```python
from build123d import *

# Parameters (mm, degrees)
SKETCH_1_W          = 120
SKETCH_1_H          = 65
EXTRUDE_1_DEPTH     = 2
EXTRUDE_2_DEPTH     = 2
SKETCH_3_R          = 2.1
CUT_EXTRUDE_1_DEPTH = 2
SKETCH_4_R          = 4
CUT_EXTRUDE_2_DEPTH = 70


with BuildPart() as part:
    # 草图1 → 凸台-拉伸1 (new body)
    with BuildSketch(Plane.XY):
        with Locations((24.994747839, 60.778264202)):
            Rectangle(SKETCH_1_W, SKETCH_1_H)
    extrude(amount=EXTRUDE_1_DEPTH)

    # 草图2 → 凸台-拉伸2 (add)
    with BuildSketch(Plane.XZ.offset(-28.278264202)):
        Polygon((-35.005252161, 2), (-35.005252161, 0), (-35.005252161, -5), (84.994747839, -28), (84.994747839, 2), align=None)
    extrude_2 = extrude(amount=EXTRUDE_2_DEPTH)

    # 镜向1: 凸台-拉伸2 across plane
    add(extrude_2.mirror(Plane.ZX.offset(60.778264202)))

    # 草图3 → 切除-拉伸1 (cut)
    with BuildSketch(Plane.XY.offset(2)):
        with Locations((-15.005252161, 80.778264202)):
            Circle(SKETCH_3_R)
        with Locations((4.994747839, 80.778264202)):
            Circle(SKETCH_3_R)
        with Locations((-15.005252161, 40.778264202)):
            Circle(SKETCH_3_R)
        with Locations((4.994747839, 40.778264202)):
            Circle(SKETCH_3_R)
    extrude(amount=-CUT_EXTRUDE_1_DEPTH, mode=Mode.SUBTRACT)

    # 草图4 → 切除-拉伸2 (cut)
    with BuildSketch(Plane(origin=(0, 26.278264202, 0), x_dir=(-1, 0, 0), z_dir=(0, -1, 0))):
        with Locations((-74.994747839, 8)):
            Circle(SKETCH_4_R)
    extrude(amount=-CUT_EXTRUDE_2_DEPTH, mode=Mode.SUBTRACT)


solid = part.part
```
Check sheet for the modelled part. Datum: model origin and axes. Units: mm. A direction names the side the tool comes from. Round coordinates to 2 decimals unless told otherwise and drop trailing zeros. Order: outer loops, then holes, each group sorted by start corner. A loop starts at its lowest first (then second) coordinate and runs counter-clockwise, first axis right, second up.
1) Mould release check, pull along Y, two halves, no side actions. Record for faces 1 (the flat face through (37, 95.278, -9)), 2 (the flat face through (84.995, 60.6, 0.3)), 3 (the flat face through (37, 28.278, -11)): +Y half, -Y half, draft (parallel to the pull), parting line (faces both ways), or undercut.
2) Section check D-D (z = -8). Record the boundary of the cut face in (x, y).
3) Scan lines: line 1 (Y direction, x = 29, z = -8.25); line 2 (Z direction, x = 15, y = 78). Record each from-to range of solid material in increasing order.
4) Tool access check on faces 4 (the flat face through (37, 93.278, -11)), 5 (the flat face through (37, 26.278, -9)). Record the directions out of +Z, -Z, +X, -X, +Y, -Y that give a thin tool (end or side, any length) a straight path to the whole face; none if there is none.
5) Go/stop test with a flat-tipped pin: pin 1 Ø12 at (y, z) = (86, -1) entering from -X. Record where the tip stops, or that it passes through.
6) Section check B-B (x = 27.5). Record the boundary of the cut face in (y, z), and give its area (3 significant figures).
7) Section check A-A (z = -25.5). Record the boundary of the cut face in (x, y).
8) Section check C-C (y = 60). Record the boundary of the cut face in (x, z), and give its area (3 significant figures).
Result:
1. face 1: +Y half
1. face 2: draft
1. face 3: undercut
2. outline: (-19.35, 26.28) - (70.99, 26.28) - (70.99, 28.28) - (-19.35, 28.28) - close; (-19.35, 93.28) - (70.99, 93.28) - (70.99, 95.28) - (-19.35, 95.28) - close; (78.99, 26.28) - (84.99, 26.28) - (84.99, 28.28) - (78.99, 28.28) - close; (78.99, 93.28) - (84.99, 93.28) - (84.99, 95.28) - (78.99, 95.28) - close
3. line 1: y = 26.28 to 28.28, 93.28 to 95.28
3. line 2: z = 0 to 2
4. face 4: -Z, +X, -X
4. face 5: +Z, -Z, +X, -X, -Y
5. pin 1: stops at x = -35.01
6. outline: (26.28, -16.98) - (28.28, -16.98) - (28.28, 0) - (93.28, 0) - (93.28, -16.98) - (95.28, -16.98) - (95.28, 2) - (26.28, 2) - close
6. area: 206 mm2
7. outline: (71.95, 26.28) - (84.99, 26.28) - (84.99, 28.28) - (71.95, 28.28) - close; (71.95, 93.28) - (84.99, 93.28) - (84.99, 95.28) - (71.95, 95.28) - close
8. outline: (-35.01, 0) - (84.99, 0) - (84.99, 2) - (-35.01, 2) - close
8. area: 240 mm2
